Job drawing, mm, ordinate dimensions from the low corner. One solid piece. A direction names the side the tool comes from. Give positions to 0.01 mm unless a question says otherwise; leave off trailing zeros. Loops run counter-clockwise (first coordinate to the right, second up) from the corner with the lowest first, then second, coordinate; pieces in that order, holes last. Notation, with made-up numbers: M -7,-20.75 L 44,-20.75 A20 cw 44,-1.75 Z; hole C 73.25,-19.75 d6. An arc over 180 degrees is marked long. Answer as CSV lines item,"result".
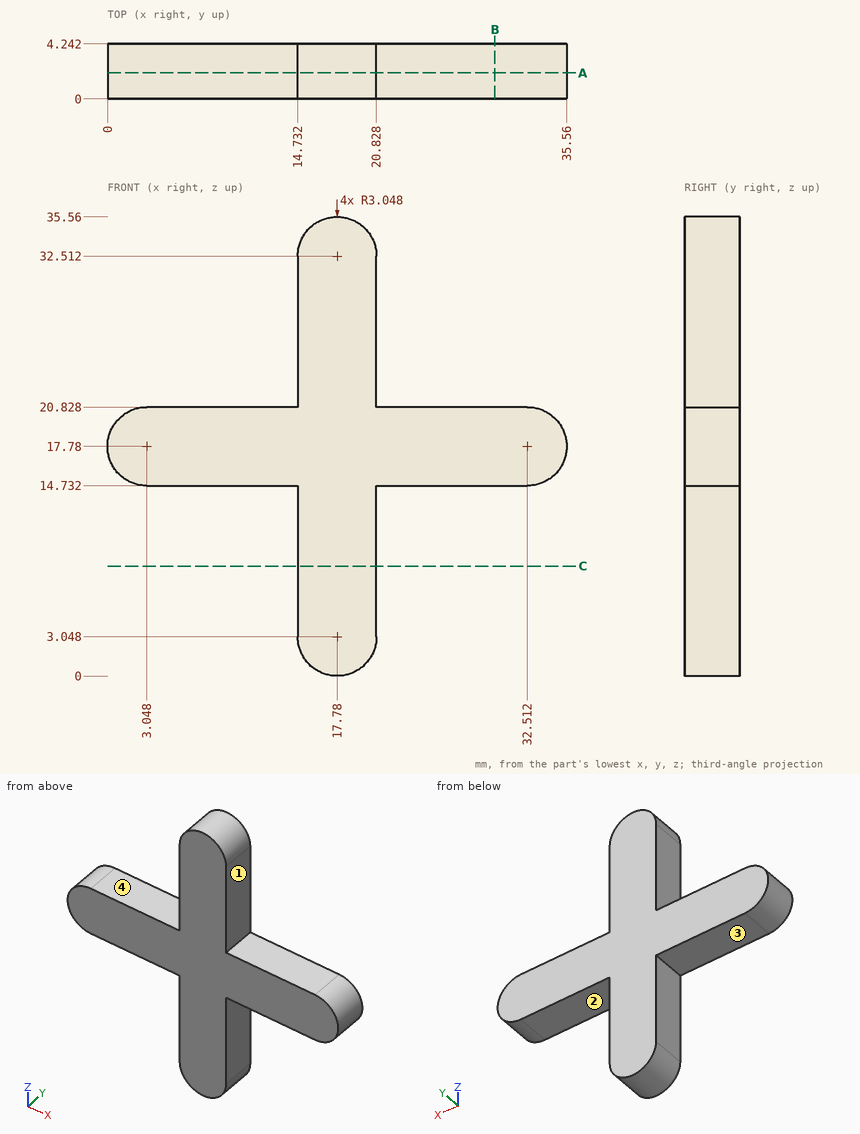
1) Band-saw the part on B-B on x = 30. Give the cut face in (y, z).
Answer below:
outline,"M 0,14.73 L 4.24,14.73 L 4.24,20.83 L 0,20.83 Z"
2) Band-saw the part on A-A on y = 2. Give the cut face in (x, z).
Answer below:
outline,"M 3.05,14.73 L 14.73,14.73 L 14.73,3.05 A3.05 ccw 20.83,3.05 L 20.83,14.73 L 32.51,14.73 A3.05 ccw 32.51,20.83 L 20.83,20.83 L 20.83,32.51 A3.05 ccw 14.73,32.51 L 14.73,20.83 L 3.05,20.83 A3.05 ccw Z"
3) Drill centre lines: line 1 (X direction, y = 1.55, z = 3); line 2 (Z direction, x = 33, y = 0.6). Where is each one in solid material? Low to high. Write a range as from..to.
Answer below:
line 1,"x = 14.73..20.83"
line 2,"z = 14.77..20.79"
4) Which spindle directions (+Z, -Z, +X, -X, +Y, -Y) get a long thin tool onto all of the face, cutting with end or side? Do the marked faces 1, 2, 3 and 4. Say none if no direction does.
Answer below:
face 1,"+Z, +X, +Y, -Y"
face 2,"-Z, +X, +Y, -Y"
face 3,"-Z, -X, +Y, -Y"
face 4,"+Z, -X, +Y, -Y"
5) Flat gauge pins, fed straight in: pin 1 (2 mm diameter, centred on y = 1, z = 9, fed in from +X); pin 2 (1.3 mm diameter, centred on y = 2, z = 7, fed in from -X); pin 3 (2 mm diameter, centred on x = 29.5, y = 1, fed in from +Z). Where does each tip first touch, or does it go through?
Answer below:
pin 1,"stops at x = 20.83"
pin 2,"stops at x = 14.73"
pin 3,"stops at z = 20.83"
6) Band-saw the part on C-C on z = 8.5. Give the cut face in (x, y).
Answer below:
outline,"M 14.73,0 L 20.83,0 L 20.83,4.24 L 14.73,4.24 Z"
